Source: CAD feature listing. Evaluate the final solid. Frame: model axes, mm. A direction names the side the tool comes from. Coordinates: 2 decimals unless noted, no trailing zeros. Write each loop counter-clockwise with the first axis right and the second up, starting at its lowest first coordinate (ties: lowest second). Pieces come first, ordered by that corner, then holes. Notation, with made-up numbers: (-40, 59) - (-21, 59) arc R8 ccw to (-21, 65) - close; hole circle Ø9 at (67, 6). An arc over 180 degrees is marked (long way). One line per item, written item: value.
Autodesk Inventor part; units mm, degrees
ref_plane "YZ Plane" through (0, 0, 0) normal (1, 0, 0) x (0, 1, 0)
ref_plane "XZ Plane" through (0, 0, 0) normal (0, 1, 0) x (-1, 0, 0)
ref_plane "XY Plane" through (0, 0, 0) normal (0, 0, 1) x (1, 0, 0)
sketch "Sketch1" plane through (0, 0, 0) normal (0, 1, 0) x (-1, 0, 0)
  line L0 (103.4541, -70.75) -> (-122.0459, -70.75)
  line L1 (-122.0459, -70.75) -> (-122.0459, 70.75)
  line L2 (-122.0459, 70.75) -> (103.4541, 70.75)
  line L3 (103.4541, 70.75) -> (103.4541, -70.75)
  line L4 (94.4541, -50.75) -> (-71.0459, -50.75)
  line L5 (-71.0459, -50.75) -> (-71.0459, 50.75)
  line L6 (-71.0459, 50.75) -> (94.4541, 50.75)
  line L7 (94.4541, 50.75) -> (94.4541, -50.75)
  line L8 (11.7041, -50.75) -> (11.7041, 50.75) construction
  line L9 (94.4541, 0) -> (-71.0459, 0) construction
  circle A0 centre (98.4541, -65.75) radius 1.75
  line L10 (103.4541, -70.75) -> (98.4541, -70.75) construction
  line L11 (98.4541, -70.75) -> (98.4541, -65.75) construction
  line L12 (98.4541, -65.75) -> (103.4541, -65.75) construction
  line L13 (103.4541, -65.75) -> (103.4541, -70.75) construction
  circle A1 centre (-117.0459, -65.75) radius 1.75
  circle A2 centre (98.4541, 65.75) radius 1.75
  circle A3 centre (-117.0459, 65.75) radius 1.75
  dimension "d0" = 101.5
  dimension "d1" = 165.5
  dimension "d3" = 20
  dimension "d4" = 3.5
  dimension "d5" = 5
  dimension "d6" = 5
  dimension "d14" = 225.5
  dimension "d16" = 9
  dimension "d21" = 5
  dimension "d22" = 5
extrude "Extrusion1" add sketch "Sketch1" along normal blind 2
sketch "Sketch2" plane through (0, 2, 0) normal (0, 1, 0) x (1, 0, 0)
  line L0 (122.0459, 70.75) -> (-103.4541, 70.75) construction
  line L1 (-103.4541, -70.75) -> (122.0459, -70.75) construction
  line L2 (-103.4541, 70.75) -> (-103.4541, -70.75) construction
  line L3 (-103.4541, 0) -> (122.0459, 0) construction
  line L4 (122.0459, -70.75) -> (122.0459, 70.75) construction
  circle A0 centre (-90.3171, 54.112) radius 1.75
  circle A1 centre (66.9089, 54.112) radius 1.75
  circle A2 centre (-90.3171, -54.112) radius 1.75
  circle A3 centre (66.9089, -54.112) radius 1.75
  line L5 (71.0459, -50.75) -> (-94.4541, -50.75) construction
  line L6 (-11.7041, -50.75) -> (-11.7041, 50.75) construction
  line L7 (-94.4541, 50.75) -> (71.0459, 50.75) construction
  point P0 (0, 0)
  dimension "d9" = 3.5
  dimension "d11" = 108.224
  dimension "d17" = 157.226
extrude "Extrusion2" cut sketch "Sketch2" against normal up to next
sketch "Sketch3" plane through (0, 2, 0) normal (0, 1, 0) x (1, 0, 0)
  circle A0 centre (-90.3171, 54.112) radius 1.75
  circle A1 centre (-90.3171, 54.112) radius 3
  line L0 (-94.4541, 50.75) -> (71.0459, 50.75) construction
  line L1 (-11.7041, 50.75) -> (-11.7041, -50.75) construction
  line L2 (71.0459, -50.75) -> (-94.4541, -50.75) construction
  line L3 (-94.4541, -50.75) -> (-94.4541, 50.75) construction
  line L4 (-94.4541, 0) -> (71.0459, 0) construction
  line L5 (71.0459, -50.75) -> (71.0459, 50.75) construction
  circle A2 centre (66.9089, 54.112) radius 3
  circle A3 centre (-90.3171, -54.112) radius 3
  circle A4 centre (66.9089, -54.112) radius 3
  circle A5 centre (-90.3171, -54.112) radius 1.75
  circle A6 centre (66.9089, -54.112) radius 1.75
  circle A7 centre (66.9089, 54.112) radius 1.75
  point P0 (0, 0)
  dimension "d18" = 6
extrude "Extrusion3" add sketch "Sketch3" against normal blind 7
properties part number "touchscreen_lid"
1) Reachability of faces 1 (the cylindrical face through (69.77, -2.46, -55.01)), 2 (the flat face through (67, -5, -52)) from +Z, -Z, +X, -X, +Y, -Y: full face, straight path, thin tool, end or side. Return the list, or none.
Values found:
face 1: -Y
face 2: +Z, -Z, +X, -X, -Y
2) Material intervals for line 1 (X direction, y = 1.3, z = 65.75); line 2 (Z direction, x = 70, y = 1); line 3 (X direction, y = 1, z = -40.5), sorted ascending.
Values found:
line 1: -103.45 to -100.2, -96.7 to 115.3, 118.8 to 122.05
line 2: -70.75 to -50.75, 50.75 to 70.75
line 3: -103.45 to -94.45, 71.05 to 122.05
3) Section query B-B on z = 44. Output: boundary loops of the cut face in (x, y), then the cut area to 3 significant figures.
Values found:
outline: (-103.45, 0) - (-94.45, 0) - (-94.45, 2) - (-103.45, 2) - close; (71.05, 0) - (122.05, 0) - (122.05, 2) - (71.05, 2) - close
area: 120 mm2
4) Section query C-C on y = -3.5. Output: boundary loops of the cut face in (x, z).
Values found:
outline: circle Ø6 at (-90.32, -54.11); circle Ø6 at (-90.32, 54.11); circle Ø6 at (66.91, -54.11); circle Ø6 at (66.91, 54.11); hole circle Ø3.5 at (-90.32, -54.11); hole circle Ø3.5 at (-90.32, 54.11); hole circle Ø3.5 at (66.91, -54.11); hole circle Ø3.5 at (66.91, 54.11)
5) Section query A-A on x = 57. Output: boundary loops of the cut face in (y, z).
Values found:
outline: (0, -70.75) - (2, -70.75) - (2, -50.75) - (0, -50.75) - close; (0, 50.75) - (2, 50.75) - (2, 70.75) - (0, 70.75) - close
6) Section query D-D on x = 105.5. Output: boundary loops of the cut face in (y, z).
Values found:
outline: (0, -70.75) - (2, -70.75) - (2, 70.75) - (0, 70.75) - close
7) Draft query along X for faces 3 (the flat face through (86, 2, 1)), 4 (the cylindrical face through (-92.698, -2.465, 55.937)). Return one class per face: released by +X, released by -X, zero draft, split by the parting line, or undercut.
Values found:
face 3: zero draft
face 4: undercut
